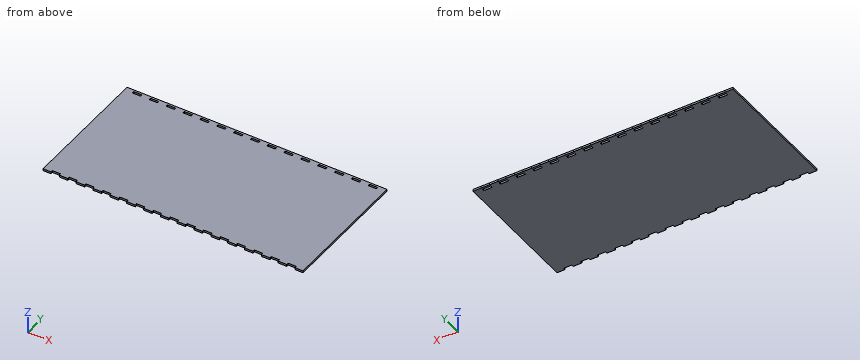
```python
from build123d import *

# Parameters (mm, degrees)
BOSS_EXTRUDE1_DEPTH      = 3.175
SKETCH2_W                = 13.407142857
SKETCH2_H                = 3.175
SKETCH2_W_2              = 12.6000002
SKETCH2_W_3              = 13.407142858
SKETCH2_W_4              = 12.6
BOSS_EXTRUDE3_DEPTH      = 3.175
BOSS_EXTRUDE3_DEPTH_BACK = 0.635
SKETCH3_W                = 3.175
SKETCH3_H                = 3.175
BOSS_EXTRUDE4_DEPTH      = 381.2


with BuildPart() as part:
    # Sketch1 → Boss-Extrude1 (new body)
    with BuildSketch(Plane.XY):
        Polygon((393.8, 203.2), (393.8, 199.925), (380.9, 199.925), (380.9, 203.2), (367.492857143, 203.2), (367.492857143, 199.925), (354.592857143, 199.925), (354.592857143, 203.2), (341.185714286, 203.2), (341.185714286, 199.925), (328.285714286, 199.925), (328.285714286, 203.2), (314.878571429, 203.2), (314.878571429, 199.925), (301.978571429, 199.925), (301.978571429, 203.2), (288.571428571, 203.2), (288.571428571, 199.925), (275.671428571, 199.925), (275.671428571, 203.2), (262.264285714, 203.2), (262.264285714, 199.925), (249.364285714, 199.925), (249.364285714, 203.2), (235.957142857, 203.2), (235.957142857, 199.925), (223.057142857, 199.925), (223.057142857, 203.2), (209.65, 203.2), (209.65, 199.925), (196.75, 199.925), (196.75, 203.2), (183.342857143, 203.2), (183.342857143, 199.925), (170.442857143, 199.925), (170.442857143, 203.2), (157.035714286, 203.2), (157.035714286, 199.925), (144.135714286, 199.925), (144.135714286, 203.2), (130.728571429, 203.2), (130.728571429, 199.925), (117.828571429, 199.925), (117.828571429, 203.2), (104.421428571, 203.2), (104.421428571, 199.925), (91.521428571, 199.925), (91.521428571, 203.2), (78.114285714, 203.2), (78.114285714, 199.925), (65.214285714, 199.925), (65.214285714, 203.2), (51.807142857, 203.2), (51.807142857, 199.925), (38.907142857, 199.925), (38.907142857, 203.2), (25.5, 203.2), (25.5, 199.925), (12.6, 199.925), (12.6000002, 203.2254), (0, 203.2254), (0, -0.0254), (12.6000002, -0.0254), (12.6, 3.275), (25.5, 3.275), (25.5, 0), (38.907142857, 0), (38.907142857, 3.275), (51.807142857, 3.275), (51.807142857, 0), (65.214285714, 0), (65.214285714, 3.275), (78.114285714, 3.275), (78.114285714, 0), (91.521428571, 0), (91.521428571, 3.275), (104.421428571, 3.275), (104.421428571, 0), (117.828571429, 0), (117.828571429, 3.275), (130.728571429, 3.275), (130.728571429, 0), (144.135714286, 0), (144.135714286, 3.275), (157.035714286, 3.275), (157.035714286, 0), (170.442857143, 0), (170.442857143, 3.275), (183.342857143, 3.275), (183.342857143, 0), (196.75, 0), (196.75, 3.275), (209.65, 3.275), (209.65, 0), (223.057142857, 0), (223.057142857, 3.275), (235.957142857, 3.275), (235.957142857, 0), (249.364285714, 0), (249.364285714, 3.275), (262.264285714, 3.275), (262.264285714, 0), (275.671428571, 0), (275.671428571, 3.275), (288.571428571, 3.275), (288.571428571, 0), (301.978571429, 0), (301.978571429, 3.275), (314.878571429, 3.275), (314.878571429, 0), (328.285714286, 0), (328.285714286, 3.275), (341.185714286, 3.275), (341.185714286, 0), (354.592857143, 0), (354.592857143, 3.275), (367.492857143, 3.275), (367.492857143, 0), (380.9, 0), (380.9, 3.275), (393.8, 3.275), (393.8, 0), (406.4, 0), (406.4, 203.2), align=None)
    extrude(amount=BOSS_EXTRUDE1_DEPTH)

    # Sketch2 → Boss-Extrude3 (add, two sides)
    with BuildSketch(Plane(origin=(0, 203.2254, 0), x_dir=(1, 0, 0), z_dir=(0, 1, 0))) as boss_extrude3_sk:
        with Locations((32.203571428, -1.5875)):
            Rectangle(SKETCH2_W, SKETCH2_H)
        with Locations((58.510714286, -1.5875)):
            Rectangle(SKETCH2_W, SKETCH2_H)
        with Locations((137.432142857, -1.5875)):
            Rectangle(SKETCH2_W, SKETCH2_H)
        with Locations((163.739285714, -1.5875)):
            Rectangle(SKETCH2_W, SKETCH2_H)
        with Locations((216.353571429, -1.5875)):
            Rectangle(SKETCH2_W, SKETCH2_H)
        with Locations((321.582142858, -1.5875)):
            Rectangle(SKETCH2_W, SKETCH2_H)
        with Locations((6.3000001, -1.5875)):
            Rectangle(SKETCH2_W_2, SKETCH2_H)
        with Locations((84.817857143, -1.5875)):
            Rectangle(SKETCH2_W, SKETCH2_H)
        with Locations((111.125, -1.5875)):
            Rectangle(SKETCH2_W_3, SKETCH2_H)
        with Locations((190.046428572, -1.5875)):
            Rectangle(SKETCH2_W, SKETCH2_H)
        with Locations((242.660714286, -1.5875)):
            Rectangle(SKETCH2_W, SKETCH2_H)
        with Locations((268.967857143, -1.5875)):
            Rectangle(SKETCH2_W, SKETCH2_H)
        with Locations((295.275, -1.5875)):
            Rectangle(SKETCH2_W_3, SKETCH2_H)
        with Locations((347.889285715, -1.5875)):
            Rectangle(SKETCH2_W, SKETCH2_H)
        with Locations((374.196428572, -1.5875)):
            Rectangle(SKETCH2_W, SKETCH2_H)
        with Locations((400.1, -1.5875)):
            Rectangle(SKETCH2_W_4, SKETCH2_H)
    extrude(amount=BOSS_EXTRUDE3_DEPTH)
    extrude(boss_extrude3_sk.sketch, amount=-BOSS_EXTRUDE3_DEPTH_BACK)

    # Sketch3 → Boss-Extrude4 (add)
    with BuildSketch(Plane(origin=(12.599987885, -7.64e-07, 0), x_dir=(0, 0, -1), z_dir=(1, -6.1e-08, 0))):
        with Locations((-1.5875, 204.812900764)):
            Rectangle(SKETCH3_W, SKETCH3_H)
    extrude(amount=BOSS_EXTRUDE4_DEPTH)


solid = part.part
```
Source: CAD feature listing. Evaluate the final solid. Frame: model axes, mm. Coordinates: 2 decimals unless noted, no trailing zeros. Order: outer loops, then holes, each group sorted by start corner. A loop starts at its lowest first (then second) coordinate and runs counter-clockwise, first axis right, second up. Notation, with made-up numbers: M 50.5,14 L 76.5,14 A28 cw 76.5,36 Z; hole C 12.25,39.25 d10. An arc over 180 degrees is marked long. Write each question's results on one line, items separated by ' | '. Start each with the question number.
1) Section query A-A (x = 124.5). Return the cut outline in (y, z) (3 decimals), plus the area to 3 significant figures.
2) Line query: line 1 (Y direction, x = 130, z = 0.4) (3 decimals); line 2 (Y direction, x = 38, z = 0.35). Output: solid intervals per line, ascending. Write a range as from..to.
3) Section query B-B (z = 1.2). Give the number of separate pieces and of enclosed holes in the cut face, plus the area to 3 significant figures.
4) Contact query for flat-ended pins moving along their axis: pin 1 Ø4 at (x, y) = (104.5, 68.5) entering from -Z; pin 2 Ø1.6 at (x, z) = (109, 1) entering from -Y; pin 3 Ø1 at (x, z) = (173.5, 2) entering from -Y (3 decimals). Output: stop coordinate, or through.
Answers:
1) outline: M 3.275,0 L 199.925,0 L 199.925,3.175 L 3.275,3.175 Z; M 203.225,0 L 206.4,0 L 206.4,3.175 L 203.225,3.175 Z | area: 634 mm^2
2) line 1: y = 3.275..199.925, 203.225..206.4 | line 2: y = 0..206.4
3) separate pieces: 1 | enclosed holes: 15 | area: 82,600 mm^2
4) pin 1: stops at z = 0 | pin 2: stops at y = 0 | pin 3: stops at y = 3.275
